Build history of the part. All positions in model axes, mm. A direction names the side the tool comes from. Round coordinates to 2 decimals unless told otherwise and drop trailing zeros. Write each loop counter-clockwise with the first axis right and the second up, starting at its lowest first coordinate (ties: lowest second). Pieces come first, ordered by that corner, then holes. Notation, with made-up numbers: (60.5, -5.5) -> (117.5, -5.5) arc R13 ccw to (117.5, 4.5) -> close; hole circle Ø8 at (79, 85). An arc over 180 degrees is marked (long way). One line per question, with ' | ' between items.
from build123d import *

# Parameters (mm, degrees)
SKETCH1_R           = 1.2
SKETCH1_R_2         = 4.4
BOSS_EXTRUDE1_DEPTH = 4
SKETCH3_W           = 34
SKETCH3_H           = 34
SKETCH3_R           = 5
SKETCH3_R_2         = 1.7
BOSS_EXTRUDE3_DEPTH = 4


with BuildPart() as part:
    # Sketch1 → Boss-Extrude1 (new body)
    with BuildSketch(Plane.XY):
        with BuildLine():
            Line((-10.25, -28.75), (10.25, -28.75))
            Line((10.25, -28.75), (10.25, 0))
            ThreePointArc((10.25, 0), (0, 10.25), (-10.25, 0))
            Line((-10.25, 0), (-10.25, -28.75))
        make_face()
        with Locations((0, 8)):
            Circle(SKETCH1_R, mode=Mode.SUBTRACT)
        with Locations((-8, 0)):
            Circle(SKETCH1_R, mode=Mode.SUBTRACT)
        with Locations((0, -8)):
            Circle(SKETCH1_R, mode=Mode.SUBTRACT)
        with Locations((8, 0)):
            Circle(SKETCH1_R, mode=Mode.SUBTRACT)
        Circle(SKETCH1_R_2, mode=Mode.SUBTRACT)
    extrude(amount=BOSS_EXTRUDE1_DEPTH)

    # Sketch3 → Boss-Extrude3 (add)
    with BuildSketch(Plane(origin=(0, -28.75, 0), x_dir=(-1, 0, 0), z_dir=(0, -1, 0))):
        with Locations((0, -17)):
            Rectangle(SKETCH3_W, SKETCH3_H)
        with Locations(Location((0, -17, 0), (0, 0, 180))):
            Circle(SKETCH3_R, mode=Mode.SUBTRACT)
        with Locations(Location((-9, -8.75, 0), (0, 0, 180))):
            Circle(SKETCH3_R_2, mode=Mode.SUBTRACT)
        with Locations(Location((9, -8.75, 0), (0, 0, 180))):
            Circle(SKETCH3_R_2, mode=Mode.SUBTRACT)
        with Locations(Location((9, -25.25, 0), (0, 0, 180))):
            Circle(SKETCH3_R_2, mode=Mode.SUBTRACT)
        with Locations(Location((-9, -25.25, 0), (0, 0, 180))):
            Circle(SKETCH3_R_2, mode=Mode.SUBTRACT)
    extrude(amount=-BOSS_EXTRUDE3_DEPTH)


solid = part.part
(1) 3-axis set-ups, long thin cutter, end or side, ignore diameter. For faces 1 (the flat face through (-10.25, -12, 2)), 2 (the flat face through (-17, -27, 17)), 3 (the flat face through (0, -11, 4)), 4 (the flat face through (10.25, -13, 2)): which of +Z, -Z, +X, -X, +Y, -Y reach the whole face in a straight line?
Calculated:
face 1: +Z, -Z, -X, +Y | face 2: +Z, -Z, -X, +Y, -Y | face 3: +Z, +X, -X, +Y | face 4: +Z, -Z, +X, +Y
(2) Wall check: line 1 (Z direction, x = -9, y = -25.9); line 2 (Y direction, x = 0, z = 2.1); line 3 (Y direction, x = 11.5, z = 24.5). Give the ranges that are in metal, low to high. Write a range as from..to.
Calculated:
line 1: 0..7.05, 10.45..23.55, 26.95..34 | line 2: -28.75..-9.2, -6.8..-4.4, 4.4..6.8, 9.2..10.25 | line 3: -28.75..-24.75
(3) Mould opens along Y. For faces 5 (the flat face through (-4, -24.75, 21)), 6 (the cylindrical face through (6.8, 0.05, 1.97)), 7 (the flat face through (17, -27, 17)) say: pulls with the +Y half, pulls with the -Y half, needs draft (parallel to the pull), parting line crosses it, or undercut.
Calculated:
face 5: pulls with the +Y half | face 6: undercut | face 7: needs draft
(4) Slice it at B-B (x = 0). Write the cut outline in (y, z).
Calculated:
outline: (-28.75, 0) -> (-9.2, 0) -> (-9.2, 4) -> (-24.75, 4) -> (-24.75, 12) -> (-28.75, 12) -> close; (-28.75, 22) -> (-24.75, 22) -> (-24.75, 34) -> (-28.75, 34) -> close; (-6.8, 0) -> (-4.4, 0) -> (-4.4, 4) -> (-6.8, 4) -> close; (4.4, 0) -> (6.8, 0) -> (6.8, 4) -> (4.4, 4) -> close; (9.2, 0) -> (10.25, 0) -> (10.25, 4) -> (9.2, 4) -> close
(5) Drop flat-ended pins along their axis: pin 1 (1.9 mm diameter, centred on x = 8, y = 0, fed in from +Z); pin 2 (5 mm diameter, centred on x = -4.5, z = 28.5, fed in from +Y); pin 3 (2 mm diameter, centred on y = -11, z = 2, fed in from +X); pin 4 (10 mm diameter, centred on x = 0.5, y = -15.5, fed in from +Z). Give the stop position or say it passes through.
Calculated:
pin 1: through | pin 2: y = -24.75 | pin 3: x = 10.25 | pin 4: z = 4
(6) Slice it at A-A (z = 21). Write the cut outline in (x, y).
Calculated:
outline: (-17, -28.75) -> (-3, -28.75) -> (-3, -24.75) -> (-17, -24.75) -> close; (3, -28.75) -> (17, -28.75) -> (17, -24.75) -> (3, -24.75) -> close
(7) Slice it at C-C (y = -8). Write the cut outline in (x, z).
Calculated:
outline: (-10.25, 0) -> (-1.2, 0) -> (-1.2, 4) -> (-10.25, 4) -> close; (1.2, 0) -> (10.25, 0) -> (10.25, 4) -> (1.2, 4) -> close
(8) Slice it at D-D (z = 8). Write the cut outline in (x, y), then the cut area to 3 significant figures.
Calculated:
outline: (-17, -28.75) -> (-10.53, -28.75) -> (-10.53, -24.75) -> (-17, -24.75) -> close; (-7.47, -28.75) -> (7.47, -28.75) -> (7.47, -24.75) -> (-7.47, -24.75) -> close; (10.53, -28.75) -> (17, -28.75) -> (17, -24.75) -> (10.53, -24.75) -> close | area: 112 mm2
